```python
from build123d import *

# Parameters (mm, degrees)
SKETCH1_W               = 63.5
SKETCH1_H               = 50.8
BOSS_EXTRUDE1_DEPTH     = 96
SKETCH2_R               = 6.35
BOSS_EXTRUDE5_DEPTH     = 36.36
SKETCH3_W               = 12.7
SKETCH3_H               = 24.13
SKETCH3_W_2             = 22.975
CUT_EXTRUDE1_DEPTH      = 64.5
SKETCH4_R               = 1.7
CUT_EXTRUDE2_DEPTH      = 2.54
MIRROR3_COPY_1_SKETCH_R = 1.7
MIRROR3_COPY_1_DEPTH    = 2.54
SKETCH5_R               = 1.7
CUT_EXTRUDE3_DEPTH      = 64.5


with BuildPart() as part:
    # Sketch1 → Boss-Extrude1 (new body)
    with BuildSketch(Plane.XY):
        Rectangle(SKETCH1_W, SKETCH1_H)
    extrude(amount=-BOSS_EXTRUDE1_DEPTH)

    # Sketch2 → Boss-Extrude5 (add)
    with BuildSketch(Plane(origin=(0, 0, -96), x_dir=(-1, 0, 0), z_dir=(0, 0, -1))):
        Circle(SKETCH2_R)
        with Locations((-19.05, 0)):
            Circle(SKETCH2_R)
        with Locations((19.05, 0)):
            Circle(SKETCH2_R)
    extrude(amount=BOSS_EXTRUDE5_DEPTH)

    # Sketch3 → Cut-Extrude1 (cut, through all)
    with BuildSketch(Plane(origin=(31.75, 0, 0), x_dir=(0, 0, -1), z_dir=(1, 0, 0))):
        with Locations((6.35, -13.335)):
            Rectangle(SKETCH3_W, SKETCH3_H)
        with Locations((84.5125, -13.335)):
            Rectangle(SKETCH3_W_2, SKETCH3_H)
    cut_extrude1 = extrude(amount=-CUT_EXTRUDE1_DEPTH, mode=Mode.SUBTRACT)

    # Mirror1: Cut-Extrude1 across plane
    add(cut_extrude1.mirror(Plane.ZX), mode=Mode.SUBTRACT)

    # Sketch4 → Cut-Extrude2 (cut)
    with BuildSketch(Plane(origin=(0, 1.27, 0), x_dir=(1, 0, 0), z_dir=(0, 1, 0))):
        with Locations((-28.4625, 79.375)):
            Circle(SKETCH4_R)
    cut_extrude2 = extrude(amount=-CUT_EXTRUDE2_DEPTH, mode=Mode.SUBTRACT)

    # Mirror2: Cut-Extrude2 across plane
    add(cut_extrude2.mirror(Plane(origin=(0, 0, 0), x_dir=(0, 0, 1), z_dir=(1, 0, 0))), mode=Mode.SUBTRACT)

    # Mirror3: Cut-Extrude2 across plane
    add(cut_extrude2.mirror(Plane(origin=(0, 0, -42.8625), x_dir=(1, 0, 0), z_dir=(0, 0, -1))), mode=Mode.SUBTRACT)

    # Mirror3 copy 1 sketch → Mirror3 copy 1 (cut)
    with BuildSketch(Plane(origin=(0, 1.27, -85.725), x_dir=(-1, 0, 0), z_dir=(0, 1, 0))):
        with Locations((-28.4625, 79.375)):
            Circle(MIRROR3_COPY_1_SKETCH_R)
    extrude(amount=-MIRROR3_COPY_1_DEPTH, mode=Mode.SUBTRACT)

    # Sketch5 → Cut-Extrude3 (cut, through all)
    with BuildSketch(Plane(origin=(31.75, 0, 0), x_dir=(0, 0, -1), z_dir=(1, 0, 0))):
        with Locations((22.826875, -11.225)):
            Circle(SKETCH5_R)
    cut_extrude3 = extrude(amount=-CUT_EXTRUDE3_DEPTH, mode=Mode.SUBTRACT)

    # Mirror4: Cut-Extrude3 across plane
    add(cut_extrude3.mirror(Plane(origin=(0, 0, -42.8625), x_dir=(1, 0, 0), z_dir=(0, 0, -1))), mode=Mode.SUBTRACT)


solid = part.part
```
Geometry check sheet. Reference: the model listing, model coordinates, mm. A direction names the side the tool comes from. Coordinates: 2 decimals unless noted, no trailing zeros. Order: outer loops, then holes, each group sorted by start corner. A loop starts at its lowest first (then second) coordinate and runs counter-clockwise, first axis right, second up.
Item 1: Depth check by flat-ended pin: pin 1 (1.5 mm diameter, centred on x = -19, z = -86, fed in from -Y); pin 2 (2 mm diameter, centred on y = -11.22, z = -22.83, fed in from +X); pin 3 (5 mm diameter, centred on x = 25, y = -13.5, fed in from +Z); pin 4 (7 mm diameter, centred on x = -13, z = -88, fed in from +Y). Enter the tip coordinate at first touch or a pass-through.
Item 2: Tool access check on faces 4 (the cylindrical face through (-24.916, -2.432, -113.925)), 5 (the flat face through (0, 1.27, -6)), 6 (the flat face through (-19, 3, -96)). Record the directions out of +Z, -Z, +X, -X, +Y, -Y that give a thin tool (end or side, any length) a straight path to the whole face; none if there is none.
Item 3: Section check A-A (z = -105). Enter the section's corners in (x, y), plus the area to 3 significant figures.
Item 4: Section check B-B (x = -19.05). Enter the section's corners in (y, z) (3 decimals).
Item 5: Section check C-C (y = 0). Count the separate pieces of the cut face and the enclosed holes in it, plus the area to 4 significant figures.
Item 6: Section check D-D (z = -85.5). Enter the section's corners in (x, y), plus the area to 3 significant figures.
Item 7: Scan lines: line 1 along Z through (x, y) = (-16.5, 4) (3 decimals); line 2 along Z through (x, y) = (8.5, 12) (3 decimals); line 3 along Y through (x, z) = (-13.5, -9). Record each from-to range of solid material in increasing order.
Item 8: Mould release check, pull along X, two halves, no side actions. Record for faces 1 (the flat face through (31.75, 0, -47)), 2 (the cylindrical face through (1.38, -6.2, -113.93)), 3 (the flat face through (0, 25.4, -42)): released by +X, released by -X, zero draft, split by the parting line, or undercut.
Check sheet entries:
1. pin 1: stops at y = -1.27
1. pin 2: passes through
1. pin 3: stops at z = -12.7
1. pin 4: stops at y = 1.27
2. face 4: -Z
2. face 5: +Z, +X, -X, +Y
2. face 6: +X, -X, +Y
3. outline: circle Ø12.7 at (-19.05, 0); circle Ø12.7 at (0, 0); circle Ø12.7 at (19.05, 0)
3. area: 380 mm2
4. outline: (-25.4, -73.025) - (-1.27, -73.025) - (-1.27, -96) - (-6.35, -96) - (-6.35, -132.36) - (6.35, -132.36) - (6.35, -96) - (1.27, -96) - (1.27, -73.025) - (25.4, -73.025) - (25.4, -12.7) - (1.27, -12.7) - (1.27, 0) - (-1.27, 0) - (-1.27, -12.7) - (-25.4, -12.7) - close; hole circle Ø3.4 at (-11.225, -62.898); hole circle Ø3.4 at (-11.225, -22.827)
5. separate pieces: 1
5. enclosed holes: 4
5. area: 7,445 mm2
6. outline: (-31.75, -1.27) - (31.75, -1.27) - (31.75, 1.27) - (-31.75, 1.27) - close
6. area: 161 mm2
7. line 1: z = -132.36 to -96, -73.025 to -12.7
7. line 2: z = -73.025 to -12.7
7. line 3: y = -1.27 to 1.27
8. face 1: released by +X
8. face 2: undercut
8. face 3: zero draft
